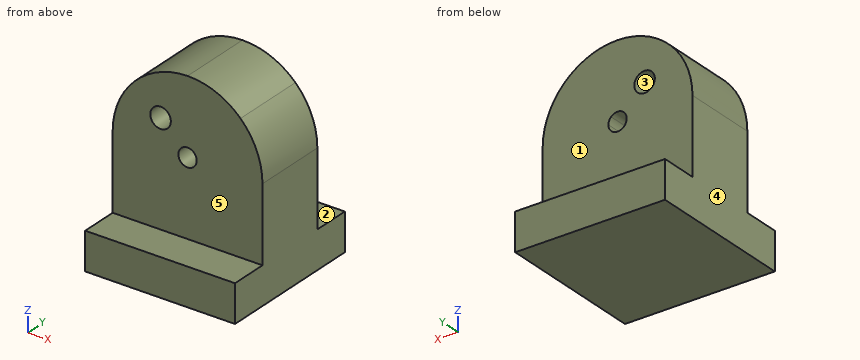
```python
from build123d import *

# Parameters (mm, degrees)
F1_DEPTH = 10
F2_R     = 2.742204369
F3_DEPTH = 25
F4_W     = 40
F4_H     = 10
F4_H_2   = 20
F5_DEPTH = 10


with BuildPart() as f1:
    # F0 (on Front) → F1 (new body, symmetric)
    with BuildSketch(Plane.XZ):
        with BuildLine():
            Line((1.7324116139, 1.7324116139), (14.1421356237, 14.1421356237))
            ThreePointArc((14.1421356237, 14.1421356237), (7.6536686307, 18.4775906571), (-3.59e-08, 20))
            ThreePointArc((-3.59e-08, 20), (-7.6536686639, 18.4775906433), (-14.1421356237, 14.1421356237))
            Line((-14.1421356237, 14.1421356237), (-1.7324116139, 1.7324116139))
            ThreePointArc((-1.7324116139, 1.7324116139), (0, 2.45), (1.7324116139, 1.7324116139))
        make_face()
        with BuildLine():
            ThreePointArc((-20, 0), (-14.1421356237, -14.1421356237), (0, -20))
            ThreePointArc((0, -20), (14.1421356237, -14.1421356237), (20, 0))
            ThreePointArc((20, 0), (18.4775906502, 7.6536686473), (14.1421356237, 14.1421356237))
            Line((14.1421356237, 14.1421356237), (1.7324116139, 1.7324116139))
            ThreePointArc((1.7324116139, 1.7324116139), (2.2635048547, 0.9375744093), (2.45, 0))
            ThreePointArc((2.45, 0), (-0.9375744093, -2.2635048547), (-1.7324116139, 1.7324116139))
            Line((-1.7324116139, 1.7324116139), (-14.1421356237, 14.1421356237))
            ThreePointArc((-14.1421356237, 14.1421356237), (-18.4775906502, 7.6536686473), (-20, 0))
        make_face()
        with BuildLine():
            Line((-20, -20), (0, -20))
            ThreePointArc((0, -20), (-14.1421356237, -14.1421356237), (-20, 0))
            Line((-20, 0), (-20, -20))
        make_face()
        with BuildLine():
            Line((0, -20), (20, -20))
            Line((20, -20), (20, 0))
            ThreePointArc((20, 0), (14.1421356237, -14.1421356237), (0, -20))
        make_face()
    extrude(amount=F1_DEPTH, both=True)

    # F2 (on face) → F3 (cut)
    with BuildSketch(Plane.XZ.offset(10)):
        with Locations((-7.2094062343, 7.4171875603)):
            Circle(F2_R)
    extrude(amount=-F3_DEPTH, mode=Mode.SUBTRACT)

    # F4 (on face) → F5 (join)
    with BuildSketch(Plane(origin=(0, 0, -20), x_dir=(1, 0, 0), z_dir=(0, 0, -1))):
        with Locations((0, 15)):
            Rectangle(F4_W, F4_H)
        Rectangle(F4_W, F4_H_2)
        with Locations((0, -15)):
            Rectangle(F4_W, F4_H)
    extrude(amount=F5_DEPTH)


solid = f1.part
```
The model under review builds one solid part; all positions refer to its coordinate system, in mm. Face numbers are marked on the shaded views. A direction names the side the tool comes from. Round coordinates to 2 decimals unless told otherwise and drop trailing zeros. Loops run counter-clockwise (first coordinate to the right, second up) from the corner with the lowest first, then second, coordinate; pieces in that order, holes last. Notation, with made-up numbers: (73, 11.5) -> (124, 11.5) arc R23 cw to (124, 39.5) -> close; hole circle Ø3 at (10.5, 47.25). An arc over 180 degrees is marked (long way). Answer as a JSON object with one key per item and string values. Group by question number.
1) We need section C-C on y = 4. Write out the cut boundary in (x, z).
2) For pin 1 Ø8 at (x, z) = (-14, 2) entering from +Y; pin 2 Ø12 at (x, y) = (-11, -12.5) entering from +Z; pin 3 Ø8 at (y, z) = (16, -2) entering from -X; pin 4 Ø3 at (x, y) = (-1.5, -17) entering from +Z, all flat-tipped, find the tip position at first contact; note any pin that passes through.
3) For the marked faces 4 and 5, list the 3-axis set-ups (+Z, -Z, +X, -X, +Y, -Y) from which the entire face can be reached by the end or side of a thin tool; tool diameter is ignored.
4) We need section D-D on z = 9. Write out the cut boundary in (x, y), then the cut area to 3 significant figures.
5) For line 1 (Z direction, x = 0, y = -3.25); line 2 (X direction, y = -3, z = 0); line 3 (Z direction, x = 14, y = 16.5), list the stretches that pass through material, from the lowest coordinate up. Write a range as [from, to].
6) We need section B-B on x = -5.5. Write out the cut boundary in (y, z).
7) Mouldability with a two-part tool opening along Z and no side actions: class the marked faces 1, 2 and 3 as released by +Z, released by -Z, zero draft, split by the parting line, or undercut.
8) We need section A-A on z = 1. Write out the cut boundary in (x, y).
Result set:
{
 "1": {"outline": "(-20, -30) -> (20, -30) -> (20, 0) arc R20 ccw to (-20, 0) -> close; hole circle Ø5.48 at (-7.21, 7.42); hole circle Ø4.9 at (0, 0)"},
 "2": {"pin 1": "y = 10", "pin 2": "z = 19.22", "pin 3": "through", "pin 4": "z = -20"},
 "3": {"face 4": "+Z, -Z, -X, +Y, -Y", "face 5": "+Z, +X, -X, -Y"},
 "4": {"outline": "(-17.86, -10) -> (-9.45, -10) -> (-9.45, 10) -> (-17.86, 10) -> close; (-4.97, -10) -> (17.86, -10) -> (17.86, 10) -> (-4.97, 10) -> close", "area": "625 mm²"},
 "5": {"line 1": "[-30, -2.45], [2.45, 20]", "line 2": "[-20, -2.45], [2.45, 20]", "line 3": "[-30, -20]"},
 "6": {"outline": "(-20, -30) -> (20, -30) -> (20, -20) -> (10, -20) -> (10, 5.27) -> (-10, 5.27) -> (-10, -20) -> (-20, -20) -> close; (-10, 9.56) -> (10, 9.56) -> (10, 19.23) -> (-10, 19.23) -> close"},
 "7": {"face 1": "zero draft", "face 2": "released by +Z", "face 3": "undercut"},
 "8": {"outline": "(-19.97, -10) -> (-2.24, -10) -> (-2.24, 10) -> (-19.97, 10) -> close; (2.24, -10) -> (19.97, -10) -> (19.97, 10) -> (2.24, 10) -> close"}
}
